Work out the finished part from the listing and answer in its coordinate system (mm). A direction names the side the tool comes from. Coordinates: 2 decimals unless noted, no trailing zeros. Order: outer loops, then holes, each group sorted by start corner. A loop starts at its lowest first (then second) coordinate and runs counter-clockwise, first axis right, second up. Notation, with made-up numbers: M 80.5,47.5 L 105.5,47.5 A26 ccw 105.5,84.5 Z; hole C 27,15.5 d3. An arc over 180 degrees is marked long. Answer in a Markdown table with one row per item. Add a question column.
Item 1: The part is cut by section C-C (y = 8). Write down the section's boundary in (x, z), then the cut area to 3 significant figures.
Item 2: Consider line 1 (X direction, y = 0.5, z = 110); line 2 (Y direction, x = 8.5, z = 83); line 3 (Y direction, x = -22, z = -5.5). Determine where each line is inside the solid, lowest interval first. Write a range as from..to.
Item 3: Flat-ended cylindrical pins translate along their axes: pin 1 Ø1 at (y, z) = (8, 65.5) entering from +X; pin 2 Ø12 at (x, z) = (-7, -57) entering from +Y; pin 3 Ø6.5 at (x, z) = (3, 99) entering from +Y. Find the tip coordinate at first contact, or state that the pin passes through.
Item 4: The part is cut by section D-D (z = 1). Write down the section's boundary in (x, y), then the cut area to 3 significant figures.
Item 5: The part is cut by section A-A (x = 0). Write down the section's boundary in (y, z).
Item 6: The mould has two halves that part along X. Classify faces 3 (the face through (0, 0, -125)), 4 (the face through (-6.503, -29.287, 1.75)), 5 (the face through (0, 27.44, -10)): released by +X, released by -X, zero draft, split by the parting line, or undercut.
Item 7: Which of the six approach directions +Z, -Z, +X, -X, +Y, -Y give full straight-line access (tool end or side, diameter ignored) to faces 1 (the face through (0, 27.44, 100)), 2 (the face through (0, 0, 125))?
Item 8: The part is cut by section B-B (z = -109). Write down the section's boundary in (x, y).
from build123d import *

# Parameters (mm, degrees)
SKETCH1_R           = 30
BOSS_EXTRUDE1_DEPTH = 125
SKETCH2_W           = 13.419524584
SKETCH2_H           = 7
CUT_EXTRUDE1_DEPTH  = 50
SKETCH3_W           = 13.419524584
SKETCH3_H           = 7
CUT_EXTRUDE2_DEPTH  = 50


with BuildPart() as part:
    # Sketch1 → Boss-Extrude1 (new, symmetric)
    with BuildSketch(Plane.XY):
        Circle(SKETCH1_R)
    extrude(amount=BOSS_EXTRUDE1_DEPTH, both=True)

    # Sketch2 → Cut-Extrude1 (cut)
    with BuildSketch(Plane.XY.offset(125)):
        with Locations((0, 30.94)):
            Rectangle(SKETCH2_W, SKETCH2_H)
    extrude(amount=-CUT_EXTRUDE1_DEPTH, mode=Mode.SUBTRACT)

    # Sketch3 → Cut-Extrude2 (cut)
    with BuildSketch(Plane.XY.offset(15)):
        with Locations((0, 30.94)):
            Rectangle(SKETCH3_W, SKETCH3_H)
    extrude(amount=-CUT_EXTRUDE2_DEPTH, mode=Mode.SUBTRACT)


solid = part.part
Reply:
| question | item | result |
|---|---|---|
| 1 | outline | M -28.91,-125 L 28.91,-125 L 28.91,125 L -28.91,125 Z |
| 1 | area | 14,500 mm2 |
| 2 | line 1 | x = -30..30 |
| 2 | line 2 | y = -28.77..28.77 |
| 2 | line 3 | y = -20.4..20.4 |
| 3 | pin 1 | stops at x = 29.05 |
| 3 | pin 2 | stops at y = 29.98 |
| 3 | pin 3 | stops at y = 27.44 |
| 4 | outline | M -6.71,27.44 L -6.71,29.24 A30 ccw long 6.71,29.24 L 6.71,27.44 Z |
| 4 | area | 2,800 mm2 |
| 5 | outline | M -30,-125 L 30,-125 L 30,-35 L 27.44,-35 L 27.44,15 L 30,15 L 30,75 L 27.44,75 L 27.44,125 L -30,125 Z |
| 6 | face 3 | zero draft |
| 6 | face 4 | split by the parting line |
| 6 | face 5 | undercut |
| 7 | face 1 | +Z, +Y |
| 7 | face 2 | +Z, +X, -X, +Y, -Y |
| 8 | outline | C 0,0 d60 |
